For this review, take the finished solid that the model builds, in its own axes (mm). Round coordinates to 2 decimals unless told otherwise and drop trailing zeros. Loops run counter-clockwise (first coordinate to the right, second up) from the corner with the lowest first, then second, coordinate; pieces in that order, holes last.
```python
from build123d import *

# Parameters (mm, degrees)
F0_W     = 20.5
F0_H     = 75
F1_DEPTH = 25
F2_R     = 8.5
F3_DEPTH = 15
F5_D     = 4.2


with BuildPart() as f1:
    # F0 (on Top) → F1 (new body)
    with BuildSketch(Plane.XY):
        with Locations((-0.3433860838, 14.475764136)):
            Rectangle(F0_W, F0_H)
    extrude(amount=F1_DEPTH)

    # F2 (on face) → F3 (join)
    with BuildSketch(Plane.XY.offset(25)):
        with Locations((0, -11.024235864)):
            Circle(F2_R)
    extrude(amount=F3_DEPTH)

    # F5 (through all)
    with Locations(Plane.XY.offset(25)):
        with Locations((-4.5289483146, 40.0326289237), (5.268279344, 40.0625547821)):
            Hole(F5_D / 2)


solid = f1.part
```
(1) Add section C-C (y = -4.5). Give the boundary of the cut face in (x, z), plus the area to 3 significant figures.
(2) Add section B-B (x = 0). Give the boundary of the cut face in (y, z).
(3) Insertion check: pin 1 Ø10 at (x, y) = (-3.5, 26.5) entering from +Z; pin 2 Ø6 at (x, z) = (2.5, 33) entering from +Y; pin 3 Ø5 at (x, z) = (-2.5, 33) entering from -Y. Each pin has a flat end and moves straight along its axis. Give the tip position at first contact, or say it passes through.
(4) Add section D-D (z = 23.5). Give the boundary of the cut face in (x, y).
(5) The part is to be moulded in two halves that separate along X. For faces 1 (the flat face through (0, -23.024, 12)), 2 (the cylindrical face through (5.542, 42.145, 12.325)), 3 (the cylindrical face through (-6.745, -16.196, 32.395)), 4 (the cylindrical face through (-5.5, 38.17, 12.33)), say which applies: pulls with the +X half, pulls with the -X half, needs draft (parallel to the pull), parting line crosses it, or undercut.
(6) Add section A-A (x = -4.25). Give the boundary of the cut face in (y, z).
(7) For L1, parallel to Y at x = 5, z = 12.5; L2, parallel to Z at x = -4.5, y = 27; L3, parallel to Y at x = -5.25, z = 16, list the stretches that pass through material, from the lowest coordinate up.
Outcome:
1. outline: (-10.59, 0) - (9.91, 0) - (9.91, 25) - (5.45, 25) - (5.45, 40) - (-5.45, 40) - (-5.45, 25) - (-10.59, 25) - close
1. area: 676 mm2
2. outline: (-23.02, 0) - (51.98, 0) - (51.98, 25) - (-2.52, 25) - (-2.52, 40) - (-19.52, 40) - (-19.52, 25) - (-23.02, 25) - close
3. pin 1: stops at z = 25
3. pin 2: stops at y = -2.52
3. pin 3: stops at y = -19.52
4. outline: (-10.59, -23.02) - (9.91, -23.02) - (9.91, 51.98) - (-10.59, 51.98) - close; hole circle Ø4.2 at (-4.53, 40.03); hole circle Ø4.2 at (5.27, 40.06)
5. face 1: needs draft
5. face 2: undercut
5. face 3: parting line crosses it
5. face 4: undercut
6. outline: (-23.02, 0) - (37.95, 0) - (37.95, 25) - (-3.66, 25) - (-3.66, 40) - (-18.39, 40) - (-18.39, 25) - (-23.02, 25) - close; (42.11, 0) - (51.98, 0) - (51.98, 25) - (42.11, 25) - close
7. L1: y = -23.02 to 37.98, 42.15 to 51.98
7. L2: z = 0 to 25
7. L3: y = -23.02 to 38.06, 42 to 51.98
